Build history of the part. All positions in model axes, mm. Face numbers are marked on the shaded views. A direction names the side the tool comes from. Round coordinates to 2 decimals unless told otherwise and drop trailing zeros. Loops run counter-clockwise (first coordinate to the right, second up) from the corner with the lowest first, then second, coordinate; pieces in that order, holes last. Notation, with made-up numbers: (58, 11.5) - (89, 11.5) arc R21 cw to (89, 43.5) - close; hole circle Ø6 at (64, 76). An arc over 180 degrees is marked (long way). Use one line per item in the form item = value. Start each with the question number.
Q1. Mould opens along X. For the marked faces 1, 2, 3 and 4 say: released by +X, released by -X, zero draft, split by the parting line, or undercut.
Q2. 3-axis set-ups, long thin cutter, end or side, ignore diameter. For the marked faces 5, 6, 7 and 8: which of +Z, -Z, +X, -X, +Y, -Y reach the whole face in a straight line?
Q3. Saw through at A-A (x = 5). Give the cut face in (y, z).
Q4. Drill centre lines: line 1 (X direction, y = -3.5, z = -27.5); line 2 (Y direction, x = -1.75, z = -17); line 3 (Y direction, x = -0.75, z = -10.5). Where is each one in solid material? Low to high.
Q5. Saw through at D-D (z = 13.5). Give the cut face in (x, y).
Q6. Saw through at B-B (z = -13). Give the cut face in (x, y).
Q7. Saw through at C-C (y = 1.5). Give the cut face in (x, z), then the cut area to 3 significant figures.
Q8. Pin check, flat tips, straight feed: pin 1 (0.7 mm diameter, centred on x = -5, z = 24.5, fed in from -Y); pin 2 (1.8 mm diameter, centred on x = -0.5, y = 0.5, fed in from -Z); pin 3 (1.5 mm diameter, centred on x = -5.5, y = 4.5, fed in from +Z). Stop position of each tip, or through.
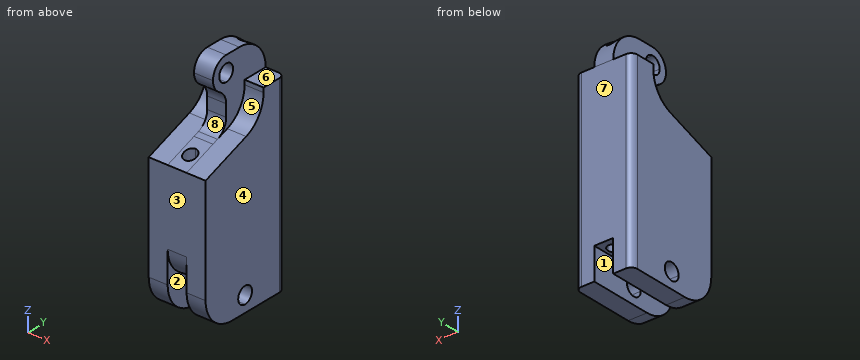
```python
from build123d import *

# Parameters (mm, degrees)
F1_DEPTH     = 15
F3_DEPTH     = 6
F5_DEPTH     = 18
F6_R         = 10
F9_DEPTH     = 6
F10_DEPTH    = 6
F11_R        = 2
F13_DEPTH    = 6
F15_R        = 10
F19_DEPTH    = 65.001
F21_DEPTH    = 60.001
F23_DEPTH    = 6
F24_T1_DEPTH = 6


# Not quite as in the source:
# - a fillet or chamfer that OpenCascade refuses, or shapes differently, is made with other operations: its cross-section is extruded or revolved along the edge and cut away or added


with BuildPart() as f1:
    # F0 (on Front) → F1 (new body, symmetric)
    with BuildSketch(Plane.XZ):
        Polygon((9, -25), (9, 25), (3, 25), (3, 35), (-3, 35), (-3, 25), (-9, 25), (-9, -25), (-9, -35), (-3, -35), (-3, -25), (3, -25), (3, -35), (9, -35), align=None)
    extrude(amount=F1_DEPTH, both=True)

    # F2 (on face) → F3 (cut)
    with BuildSketch(Plane(origin=(-3, 0, 0), x_dir=(0, -1, 0), z_dir=(-1, 0, 0))):
        with BuildLine():
            ThreePointArc((0, 32.62), (-2.62, 30), (0, 27.38))
            Line((0, 27.38), (0, 32.62))
        make_face()
        with BuildLine():
            Line((0, 32.62), (0, 27.38))
            ThreePointArc((0, 27.38), (1.8526197667, 28.1473802333), (2.62, 30))
            ThreePointArc((2.62, 30), (1.8526197667, 31.8526197667), (0, 32.62))
        make_face()
    extrude(amount=-F3_DEPTH, mode=Mode.SUBTRACT)

    # F4 (on face) → F5 (cut)
    with BuildSketch(Plane(origin=(-9, 0, 0), x_dir=(0, -1, 0), z_dir=(-1, 0, 0))):
        with BuildLine():
            ThreePointArc((0, -32.62), (1.8526197667, -31.8526197667), (2.62, -30))
            ThreePointArc((2.62, -30), (-1.8526197667, -28.1473802333), (0, -32.62))
        make_face()
    extrude(amount=-F5_DEPTH, mode=Mode.SUBTRACT)

    # F6
    f6_edges = [f1.edges().sort_by_distance(p)[0] for p in [
        (0, 15, 35),
        (0, -15, 35),
        (6, -15, -35),
        (-6, -15, -35),
    ]]
    fillet(f6_edges, radius=F6_R)

    # F8 (on face) → F9 (cut)
    with BuildSketch(Plane(origin=(-9, 0, 0), x_dir=(0, -1, 0), z_dir=(-1, 0, 0))):
        with BuildLine():
            ThreePointArc((-7, 23.5872004348), (-5.1915204429, 17.8514360713), (-0.4202014333, 14.190274227))
            Line((-0.4202014333, 14.190274227), (15, 8.5777798989))
            Line((15, 8.5777798989), (15, 25))
            Line((15, 25), (-7, 25))
            Line((-7, 25), (-7, 23.5872004348))
        make_face()
    extrude(amount=-F9_DEPTH, mode=Mode.SUBTRACT)

    # F7 (on face) → F10 (cut)
    with BuildSketch(Plane.YZ.offset(9)):
        with BuildLine():
            Line((7, 25), (-15, 25))
            Line((-15, 25), (-15, 8.57778))
            Line((-15, 8.57778), (0.4202014333, 14.1902743281))
            ThreePointArc((0.4202014333, 14.1902743281), (5.1915204429, 17.8514361724), (7, 23.587200536))
            Line((7, 23.587200536), (7, 25))
        make_face()
    extrude(amount=-F10_DEPTH, mode=Mode.SUBTRACT)

    # F11
    f11_edges = [f1.edges().sort_by_distance(p)[0] for p in [
        (9, 15, -5),
        (-9, 15, -5),
    ]]
    fillet(f11_edges, radius=F11_R)

    # F12 (on face) → F13 (cut)
    with BuildSketch(Plane(origin=(-3, 0, 0), x_dir=(0, -1, 0), z_dir=(-1, 0, 0))):
        with BuildLine():
            Line((5, 35), (0, 35))
            ThreePointArc((0, 35), (3.5355339059, 33.5355339059), (5, 30))
            Line((5, 30), (5, 12.2174822415))
            Line((5, 12.2174822415), (15, 8.5777798989))
            Line((15, 8.5777798989), (15, 25))
            ThreePointArc((15, 25), (12.0710678119, 32.0710678119), (5, 35))
        make_face()
    extrude(amount=-F13_DEPTH, mode=Mode.SUBTRACT)

    # F15
    f15_edges = [f1.edges().sort_by_distance(p)[0] for p in [
        (0, -15, -25),
    ]]
    fillet(f15_edges, radius=F15_R)

    # F18 (on face) → F19 (cut, through all)
    with BuildSketch(Plane.XY.offset(30)):
        with BuildLine():
            ThreePointArc((2, -10), (1.4142135624, -8.5857864376), (0, -8))
            Line((0, -8), (0, -12))
            ThreePointArc((0, -12), (1.4142135624, -11.4142135624), (2, -10))
        make_face()
        with BuildLine():
            Line((0, -12), (0, -8))
            ThreePointArc((0, -8), (-2, -10), (0, -12))
        make_face()
    extrude(amount=-F19_DEPTH, mode=Mode.SUBTRACT)

    # F20 (on face) → F21 (cut, through all)
    with BuildSketch(Plane(origin=(0, 0, -25), x_dir=(1, 0, 0), z_dir=(0, 0, -1))):
        with BuildLine():
            ThreePointArc((0, -9), (-2, -11), (0, -13))
            Line((0, -13), (0, -11))
            Line((0, -11), (0, -9))
        make_face()
        with BuildLine():
            Line((0, -11), (0, -13))
            ThreePointArc((0, -13), (1.4142135624, -12.4142135624), (2, -11))
            ThreePointArc((2, -11), (1.4142135624, -9.5857864376), (0, -9))
            Line((0, -9), (0, -11))
        make_face()
    extrude(amount=-F21_DEPTH, mode=Mode.SUBTRACT)

    # F22 (on face) → F23 (cut)
    with BuildSketch(Plane.YZ.offset(3)):
        with BuildLine():
            ThreePointArc((0, 25), (-3.5355339059, 26.4644660941), (-5, 30))
            Line((-5, 30), (-5, 12.2174822415))
            Line((-5.0000000325, 12.2174823308), (0, 14.037333514))
            Line((0, 14.037333514), (0, 25))
        make_face()
    extrude(amount=-F23_DEPTH, mode=Mode.SUBTRACT)

    # F24: fillet of radius 5 on 2 edges, made by hand

    # F24_s2 → F24_t1 (join)
    with BuildSketch(Plane.YZ.offset(-3)):
        with BuildLine():
            ThreePointArc((-2.5, 25.6698729811), (-0.6698729811, 23.8397459622), (0, 21.3397459622))
            Line((0, 21.3397459622), (0, 25))
            ThreePointArc((0, 25), (-1.2940952255, 25.1703708686), (-2.5, 25.6698729811))
        make_face()
        with BuildLine():
            ThreePointArc((-3.2898992834, 12.8399081011), (-0.9042397786, 14.6704890233), (0, 17.538371205))
            Line((0, 17.538371205), (0, 14.037333514))
            Line((0, 14.037333514), (-3.2898992834, 12.8399081011))
        make_face()
    extrude(amount=F24_T1_DEPTH)


solid = f1.part
```
Report:
q1.face_1 = undercut
q1.face_2 = undercut
q1.face_3 = zero draft
q1.face_4 = released by +X
q2.face_5 = +Z, +X, -Y
q2.face_6 = +Z, +X, +Y, -Y
q2.face_7 = +Z, -Z, +X, -X, +Y
q2.face_8 = +X, -X, -Y
q3.outline = (-15, -25) arc R10 ccw to (-5, -35) - (15, -35) - (15, 25) - (7, 25) - (7, 23.59) arc R10 cw to (0.42, 14.19) - (-15, 8.58) - close; hole circle Ø5.24 at (0, -30)
q4.line_1 = -9 to -3, 3 to 9
q4.line_2 = -14.8 to -10.97, -9.03 to 10.03, 11.97 to 15
q4.line_3 = -15 to -11.85, -8.15 to 9.15, 12.85 to 15
q5.outline = (-9, -1.48) - (-3, -1.48) - (-3, -2.05) - (3, -2.05) - (3, -1.48) - (9, -1.48) - (9, 13) arc R2 ccw to (7, 15) - (-7, 15) arc R2 ccw to (-9, 13) - close; hole circle Ø4 at (0, 11)
q6.outline = (-9, -15) - (9, -15) - (9, 13) arc R2 ccw to (7, 15) - (-7, 15) arc R2 ccw to (-9, 13) - close; hole circle Ø4 at (0, -10); hole circle Ø4 at (0, 11)
q7.outline = (-9, -35) - (-3, -35) - (-3, -32.15) - (-9, -32.15) - close; (-9, -27.85) - (-3, -27.85) - (-3, -25) - (3, -25) - (3, -27.85) - (9, -27.85) - (9, 14.66) - (3, 14.66) - (3, 27.85) - (-3, 27.85) - (-3, 14.66) - (-9, 14.66) - close; (-3, 32.15) - (3, 32.15) - (3, 35) - (-3, 35) - close; (3, -35) - (9, -35) - (9, -32.15) - (3, -32.15) - close
q7.area = 879 mm²
q8.pin_1 = 7
q8.pin_2 = -25
q8.pin_3 = 17.94
